Geometry check sheet. Reference: the model listing, model coordinates, mm. Coordinates: 2 decimals unless noted, no trailing zeros. Write each loop counter-clockwise with the first axis right and the second up, starting at its lowest first coordinate (ties: lowest second). Pieces come first, ordered by that corner, then holes. Notation, with made-up numbers: (75.25, 83) -> (81.25, 83) arc R26 cw to (81.25, 119) -> close; hole circle Ø5 at (-6, -27). An arc over 180 degrees is marked (long way). Answer in a Markdown table with one row per item. Add a question column.
Q1. Thickness scan on line 1 (Y direction, x = 6, z = 0.95); line 2 (Y direction, x = -1, z = 0.25); line 3 (X direction, y = 143, z = 1.9). Record the ranges inside material, lowest first.
Q2. Section check B-B, the plane y = 126.5. Record the boundary of the cut face in (x, z), and give its area (3 significant figures).
Q3. Section check C-C, the plane z = 1.75. Count the separate pieces of the cut face and the enclosed holes in it, and give its area (3 significant figures).
Q4. Gauge pin test, flat end, axial feed: P1, Ø1.5, axis at y = -37, z = 2, coming from the -X side. Record the tip position at first contact, or that the pin passes through.
Q5. Section check A-A, the plane x = -125.5. Record the boundary of the cut face in (y, z), and give its area (3 significant figures).
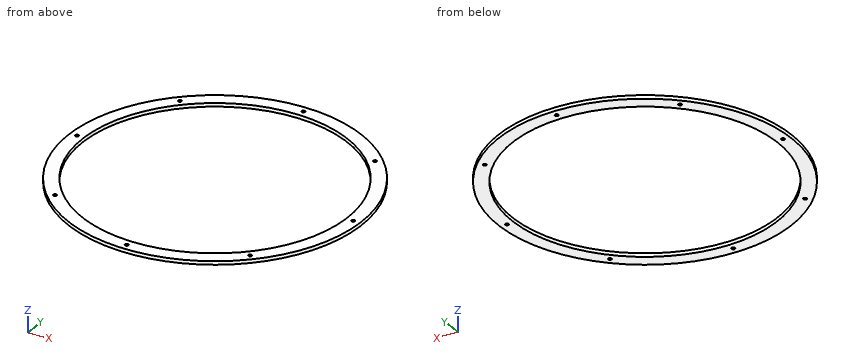
```python
from build123d import *

# Parameters (mm, degrees)
SKETCH1_R           = 210
SKETCH1_R_2         = 190
BOSS_EXTRUDE1_DEPTH = 5
M6_TAPPED_HOLE1_D   = 5
CIRPATTERN1_COUNT   = 8


with BuildPart() as part:
    # Sketch1 → Boss-Extrude1 (new body)
    with BuildSketch(Plane.XY):
        Circle(SKETCH1_R)
        Circle(SKETCH1_R_2, mode=Mode.SUBTRACT)
    extrude(amount=BOSS_EXTRUDE1_DEPTH)

    # M6 Tapped Hole1 (through all)
    with Locations(Plane.XY.offset(5)):
        with Locations((0, 200)):
            m6_tapped_hole1 = Hole(M6_TAPPED_HOLE1_D / 2)

    # CirPattern1: M6 Tapped Hole1 ×8 about axis
    cirpattern1_axis = Axis((0, 0, 0), (0, 0, 1))
    for i in range(1, CIRPATTERN1_COUNT):
        add(m6_tapped_hole1.rotate(cirpattern1_axis, i * 360 / CIRPATTERN1_COUNT), mode=Mode.SUBTRACT)


solid = part.part
```
Calculated:
| question | item | result |
|---|---|---|
| 1 | line 1 | y = -209.91 to -189.91, 189.91 to 209.91 |
| 1 | line 2 | y = -210 to -202.29, -197.71 to -190, 190 to 197.71, 202.29 to 210 |
| 1 | line 3 | x = -153.79 to -143.36, -139.48 to -125.1, 125.1 to 139.48, 143.36 to 153.79 |
| 2 | outline | (-167.62, 0) -> (-141.77, 0) -> (-141.77, 5) -> (-167.62, 5) -> close; (141.77, 0) -> (167.62, 0) -> (167.62, 5) -> (141.77, 5) -> close |
| 2 | area | 259 mm² |
| 3 | separate pieces | 1 |
| 3 | enclosed holes | 9 |
| 3 | area | 25,000 mm² |
| 4 | P1 | stops at x = -206.85 |
| 5 | outline | (-168.37, 0) -> (-142.65, 0) -> (-142.65, 5) -> (-168.37, 5) -> close; (142.65, 0) -> (168.37, 0) -> (168.37, 5) -> (142.65, 5) -> close |
| 5 | area | 257 mm² |
